```python
from build123d import *

# Parameters (mm, degrees)
PAD_DEPTH       = 450
POCKET_DEPTH    = 669.832754
POCKET001_DEPTH = 669.832754
PAD001_DEPTH    = 50
PAD002_DEPTH    = 200
POCKET002_DEPTH = 446.248375


with BuildPart() as part:
    # Sketch → Pad (new body)
    with BuildSketch(Plane.YZ):
        Polygon((0, 0), (-93.755817, 693.692905), (-413.044342, 693.692905), (-669.831754, 0), (-631.063619, 0), (-369.641988, 644.527666), (-143.466095, 644.527666), (-31.204716, 0), align=None)
    extrude(amount=PAD_DEPTH)

    # Sketch001 → Pocket (cut, through all)
    with BuildSketch(Plane.XZ):
        Polygon((0, 0), (68.653915, 756.659241), (-58.010685, 756.659241), (-58.010685, 0), align=None)
        Polygon((446.247375, 0), (380.038452, 758.557922), (486.73526, 758.557922), (486.73526, 0), align=None)
    extrude(amount=POCKET_DEPTH, mode=Mode.SUBTRACT)

    # Sketch002 → Pocket001 (cut, through all)
    with BuildSketch(Plane.XZ):
        Polygon((15.741308, -101.116302), (87.504074, 629.326477), (348.92572, 629.326477), (430.940308, -101.116302), align=None)
    extrude(amount=POCKET001_DEPTH, mode=Mode.SUBTRACT)

    # Sketch003 (on Face2 of Pocket001) → Pad001 (join)
    with BuildSketch(Plane(origin=(0, 0, 693.692905), x_dir=(0, -1, 0), z_dir=(0, 0, 1))):
        with BuildLine():
            ThreePointArc((186.040695, 396.127842), (13.348888, 223.436035), (186.040695, 50.744228))
            Line((186.040695, 50.744228), (371.77124, 50.744228))
            ThreePointArc((371.77124, 50.744228), (544.463047, 223.436035), (371.77124, 396.127842))
            Line((186.040695, 396.127842), (371.77124, 396.127842))
        make_face()
    extrude(amount=PAD001_DEPTH)

    # Sketch004 (on Face22 of Pad001) → Pad002 (join)
    with BuildSketch(Plane(origin=(0, 0, 743.692905), x_dir=(0, -1, 0), z_dir=(0, 0, 1))):
        with BuildLine():
            ThreePointArc((415.269303, 61.142208), (533.592428, 226.236558), (415.268147, 391.330079))
            Line((415.268147, 391.330079), (199.105545, 391.330079))
            Line((199.105545, 391.330079), (199.105545, 347.998))
            Line((199.105545, 347.998), (397.824581, 347.998))
            ThreePointArc((400.528442, 105.363647), (486.971795, 227.659194), (397.824581, 347.998))
            Line((400.528442, 105.363647), (196.068253, 105.363647))
            Line((196.068253, 105.363647), (196.068253, 61.142208))
            Line((196.068253, 61.142208), (415.269303, 61.142208))
        make_face()
    extrude(amount=PAD002_DEPTH)

    # Sketch006 → Pocket002 (cut, through all)
    with BuildSketch(Plane.YZ):
        Polygon((-193.693634, 744.098999), (-545.720642, 1034.452026), (-176.155548, 1034.452026), (-176.155548, 744.098999), align=None)
    extrude(amount=POCKET002_DEPTH, mode=Mode.SUBTRACT)


solid = part.part
```
Source: CAD feature listing. Evaluate the final solid. Frame: model axes, mm. A direction names the side the tool comes from. Round coordinates to 2 decimals unless told otherwise and drop trailing zeros. Loops run counter-clockwise (first coordinate to the right, second up) from the corner with the lowest first, then second, coordinate; pieces in that order, holes last. Notation, with made-up numbers: M -1.75,-19.5 L 2.25,-19.5 A31 cw 2.25,6.5 Z; hole C 32.5,11.5 d7. An arc over 180 degrees is marked long. Use a Markdown table: item, result. Add a question column.
1. Section query B-B on y = -597.5. Return the cut outline in (x, z), then the cut area to 3 significant figures.
2. Section query D-D on y = -234.5. Return the cut outline in (x, z).
3. Section query A-A on z = 76.5. Return the cut outline in (x, y).
4. Mould query, pull axis Z, two halves, no side actions, for faces 4 (the flat face through (224, -426, 693.693)), 5 (the flat face through (13, -16, 0)), 6 (the flat face through (105.364, -322, 809)), 7 (the flat face through (370.83, -60.55, 448)). Classes: pulls with the +Z half, pulls with the -Z half, needs draft (parallel to the pull), parting line crosses it, or undercut.
5. Line query: line 1 (X direction, y = -354.5, z = 765); line 2 (Z direction, x = 155, y = -126); line 3 (Z direction, x = 298, y = -162.5). Output: solid intervals per line, ascending.
6. Reachability of faces 1 (the flat face through (61.142, -328, 814)), 2 (the flat face through (58.735, -70.081, 336.503)), 3 (the cylindrical face through (227.23, -13.39, 718.34)) from +Z, -Z, +X, -X, +Y, -Y: full face, straight path, thin tool, end or side. Return the list, or none.
7. Contact query for flat-ended pins moving along their axis: P1, Ø4, axis at x = 197, y = -352.5, coming from the -Z side; P2, Ø18.5, axis at x = 173, y = -404, coming from the -Z side; P3, Ø1.8, axis at x = 389.5, y = -419, coming from the -Z side. Output: stop coordinate, or through.
8. Section query C-C on x = 238. Return the cut outline in (y, z).
Reported:
| question | item | result |
|---|---|---|
| 1 | outline | M 7.51,82.75 L 33.81,82.75 L 44.87,195.4 L 17.73,195.4 Z; M 397.65,195.4 L 410.3,82.75 L 439.02,82.75 L 429.19,195.4 Z |
| 1 | area | 6,400 mm² |
| 2 | outline | M 50.74,693.69 L 62.94,693.69 L 58.48,644.53 L 389.99,644.53 L 385.7,693.69 L 396.13,693.69 L 396.13,743.69 L 391.33,743.69 L 391.33,777.76 L 348,777.76 L 348,743.69 L 105.36,743.69 L 105.36,777.76 L 61.14,777.76 L 61.14,743.69 L 50.74,743.69 Z |
| 3 | outline | M 6.94,-641.51 L 33.19,-641.51 L 33.19,-600.04 L 6.94,-600.04 Z; M 6.94,-44.53 L 33.19,-44.53 L 33.19,-10.34 L 6.94,-10.34 Z; M 411,-641.51 L 439.57,-641.51 L 439.57,-600.04 L 411,-600.04 Z; M 411,-44.53 L 439.57,-44.53 L 439.57,-10.34 L 411,-10.34 Z |
| 4 | face 4 | undercut |
| 4 | face 5 | pulls with the -Z half |
| 4 | face 6 | needs draft |
| 4 | face 7 | undercut |
| 5 | line 1 | x = 61.14 to 105.36, 348 to 391.33 |
| 5 | line 2 | z = 629.33 to 743.69 |
| 5 | line 3 | z = 644.53 to 743.69 |
| 6 | face 1 | +Z, -X, +Y, -Y |
| 6 | face 2 | -Z, +Y, -Y |
| 6 | face 3 | +Z, +Y |
| 7 | P1 | stops at z = 644.53 |
| 7 | P2 | stops at z = 629.33 |
| 7 | P3 | stops at z = 520.62 |
| 8 | outline | M -543.85,693.69 L -413.04,693.69 L -436.87,629.33 L -375.81,629.33 L -369.64,644.53 L -143.47,644.53 L -140.82,629.33 L -85.06,629.33 L -93.76,693.69 L -13.96,693.69 L -13.96,743.69 L -486.44,743.69 L -486.44,943.69 L -533.2,943.69 L -533.2,743.69 L -543.85,743.69 Z |
